Source: CAD feature listing. Evaluate the final solid. Frame: model axes, mm. Face numbers are marked on the shaded views. A direction names the side the tool comes from. Round coordinates to 2 decimals unless told otherwise and drop trailing zeros. Loops run counter-clockwise (first coordinate to the right, second up) from the corner with the lowest first, then second, coordinate; pieces in that order, holes last. Notation, with made-up numbers: M 5.5,34.25 L 52.5,34.25 A9 cw 52.5,39.25 Z; hole C 64,-19 d5. An arc over 180 degrees is marked long. One line per item, written item: value.
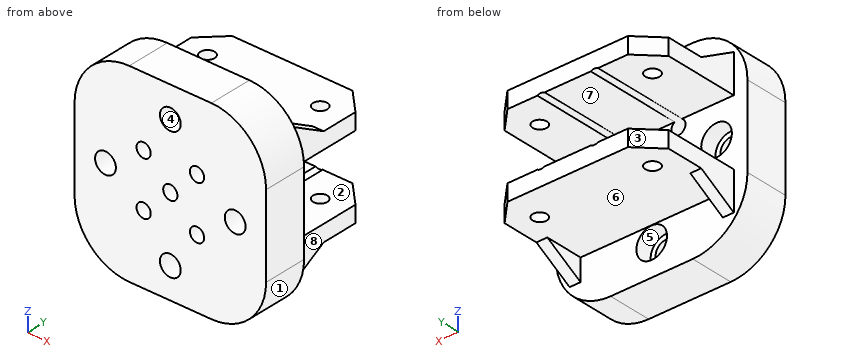
from build123d import *

# Parameters (mm, degrees)
SKETCH_2_R          = 1.3
EXTRUDE_1_DEPTH     = 9
SKETCH_3_W          = 30
SKETCH_3_H          = 20.835575778
CUT_EXTRUDE_1_DEPTH = 6
EXTRUDE_START       = -6.7
EXTRUDE_2_DEPTH     = 8
CUT_EXTRUDE_START   = -14.7
SKETCH_5_R          = 1.3
SKETCH_5_R_2        = 1.9
CUT_EXTRUDE_2_DEPTH = 30
EXTRUDE_3_DEPTH     = 2
EXTRUDE_4_DEPTH     = 2
SKETCH_11_R         = 2.8
CUT_EXTRUDE_3_DEPTH = 3


with BuildPart() as part:
    # 草图2 → 凸台-拉伸1 (new, symmetric)
    with BuildSketch(Plane.XY):
        Polygon((-11, 11), (11, 11), (15, 7), (15, -11), (-15, -11), (-15, 7), align=None)
        with Locations((-10.3, 5)):
            Circle(SKETCH_2_R, mode=Mode.SUBTRACT)
        with Locations(Location((10.3, 5, 0), (0, 0, 180))):
            Circle(SKETCH_2_R, mode=Mode.SUBTRACT)
    extrude(amount=EXTRUDE_1_DEPTH, both=True)

    # 草图3 → 切除-拉伸1 (cut, symmetric)
    with BuildSketch(Plane.XY):
        with Locations((0, 3.717787889)):
            Rectangle(SKETCH_3_W, SKETCH_3_H)
    extrude(amount=CUT_EXTRUDE_1_DEPTH, both=True, mode=Mode.SUBTRACT)

    # 草图6 → 凸台-拉伸2 (add)
    with BuildSketch(Plane(origin=(0, 0, 0), x_dir=(1, 0, 0), z_dir=(0, 1, 0)).offset(EXTRUDE_START)):
        with BuildLine():
            Line((-7.5, -17.5), (7.5, -17.5))
            ThreePointArc((7.5, -17.5), (14.571067812, -14.571067812), (17.5, -7.5))
            Line((17.5, -7.5), (17.5, 7.5))
            ThreePointArc((17.5, 7.5), (14.571067812, 14.571067812), (7.5, 17.5))
            Line((7.5, 17.5), (-7.5, 17.5))
            ThreePointArc((-7.5, 17.5), (-14.571067812, 14.571067812), (-17.5, 7.5))
            Line((-17.5, 7.5), (-17.5, -7.5))
            ThreePointArc((-17.5, -7.5), (-14.571067812, -14.571067812), (-7.5, -17.5))
        make_face()
    extrude(amount=-EXTRUDE_2_DEPTH)

    # 草图5 → 切除-拉伸2 (cut)
    with BuildSketch(Plane(origin=(0, 0, 0), x_dir=(1, 0, 0), z_dir=(0, 1, 0)).offset(CUT_EXTRUDE_START)):
        with Locations(Location((0, 0, 0), (0, 0, 90))):
            Circle(SKETCH_5_R)
        with Locations(Location((-4.87903679, 4.87903679, 0), (0, 0, 90))):
            Circle(SKETCH_5_R)
        with Locations(Location((-11.85, 0, 0), (0, 0, 90))):
            Circle(SKETCH_5_R_2)
        with Locations(Location((0, 11.85, 0), (0, 0, 90))):
            Circle(SKETCH_5_R_2)
        with Locations(Location((4.87903679, 4.87903679, 0), (0, 0, 90))):
            Circle(SKETCH_5_R)
        with Locations(Location((11.85, 0, 0), (0, 0, 90))):
            Circle(SKETCH_5_R_2)
        with Locations(Location((4.87903679, -4.87903679, 0), (0, 0, 90))):
            Circle(SKETCH_5_R)
        with Locations(Location((0, -11.85, 0), (0, 0, 90))):
            Circle(SKETCH_5_R_2)
        with Locations(Location((-4.87903679, -4.87903679, 0), (0, 0, 90))):
            Circle(SKETCH_5_R)
    extrude(amount=CUT_EXTRUDE_2_DEPTH, mode=Mode.SUBTRACT)

    # 草图7 → 凸台-拉伸3 (add)
    with BuildSketch(Plane(origin=(15, 0, 0), x_dir=(0, 0, -1), z_dir=(1, 0, 0))):
        Polygon((-9, 0.3), (-13, -6.7), (-9, -6.7), align=None)
        Polygon((9, -6.7), (9, 0.3), (13, -6.7), align=None)
    extrude(amount=-EXTRUDE_3_DEPTH)

    # 草图10 → 凸台-拉伸4 (add)
    with BuildSketch(Plane.ZY.offset(15)):
        Polygon((-9, 0.15), (-13, -6.7), (-9, -6.7), align=None)
        Polygon((9, -6.7), (9, 0.15), (13, -6.7), align=None)
    extrude(amount=-EXTRUDE_4_DEPTH)

    # 草图11 → 切除-拉伸3 (cut)
    with BuildSketch(Plane(origin=(0, -6.7, 0), x_dir=(1, 0, 0), z_dir=(0, 1, 0))):
        with Locations(Location((0, 11.85, 0), (0, 0, 270))):
            Circle(SKETCH_11_R)
        with Locations(Location((11.85, 0, 0), (0, 0, 270))):
            Circle(SKETCH_11_R)
        with Locations(Location((0, -11.85, 0), (0, 0, 270))):
            Circle(SKETCH_11_R)
        with Locations(Location((-11.85, 0, 0), (0, 0, 270))):
            Circle(SKETCH_11_R)
    extrude(amount=-CUT_EXTRUDE_3_DEPTH, mode=Mode.SUBTRACT)


solid = part.part
1. Section query C-C (x = -7). Return the cut outline in (y, z).
Report:
outline: M -14.7,-17.5 L -6.7,-17.5 L -6.7,-9 L 11,-9 L 11,-6 L -6.7,-6 L -6.7,6 L 11,6 L 11,9 L -6.7,9 L -6.7,17.5 L -14.7,17.5 Z
2. Pin query (flat end, axial travel): pin 1 (4.5 mm diameter, centred on x = 11.5, y = 6.5, fed in from -Z); pin 2 (3.5 mm diameter, centred on x = -10.3, y = 5, fed in from +Z); pin 3 (9 mm diameter, centred on x = 0, z = 11.85, fed in from +Y); pin 4 (4.5 mm diameter, centred on y = -2, z = 10.5, fed in from -X). Return the tip coordinate at first contact, or that it passes through.
Report:
pin 1: stops at z = -9
pin 2: stops at z = 9
pin 3: stops at y = 11
pin 4: stops at x = -15
3. Reachability of the marked faces 5, 6, 7 and 8 from +Z, -Z, +X, -X, +Y, -Y: full face, straight path, thin tool, end or side. Return the list, or none.
Report:
face 5: +Y
face 6: -Z, +Y
face 7: +X, -X, +Y
face 8: +Z, -Z, +X, +Y
4. Pull-direction query (Z, two-part tool) for the marked faces 1, 2, 3 and 4; classes: released by +Z, released by -Z, zero draft, split by the parting line, or undercut.
Report:
face 1: released by -Z
face 2: undercut
face 3: zero draft
face 4: undercut
5. Section query A-A (y = 5). Count the separate pieces of the cut face and the enclosed holes in it, and give its area (3 significant figures).
Report:
separate pieces: 6
enclosed holes: 0
area: 148 mm2
6. Ray query, line 1 (Z direction, x = -6.5, y = 9); line 2 (X direction, y = -7.35, z = 0); line 3 (Z direction, x = -4, y = -9.75). Return the intervals inside material, ascending. Write a range as [from, to].
Report:
line 1: z = [-9, -6], [6, 9]
line 2: x = [-17.5, -14.65], [-9.05, -1.3], [1.3, 9.05], [14.65, 17.5]
line 3: z = [-17.5, -5.84], [-3.92, 3.92], [5.84, 17.5]
